For this review, take the finished solid that the model builds, in its own axes (mm). Face numbers are marked on the shaded views. A direction names the side the tool comes from. Coordinates: 2 decimals unless noted, no trailing zeros. Order: outer loops, then holes, each group sorted by start corner. A loop starts at its lowest first (then second) coordinate and runs counter-clockwise, first axis right, second up. Notation, with made-up numbers: (46.5, 30.25) -> (62.5, 30.25) arc R21 cw to (62.5, 51.25) -> close; hole circle Ø1 at (3, -19). An arc over 180 degrees is marked (long way). Return JSON: item names as keys, results as strings. Group by question number.
Item 1: Machinability: for the marked faces 5, 6 and 7, which of the approach directions +Z, -Z, +X, -X, +Y, -Y give a long, thin tool a straight path to every point of the face, cutting with its end or side? Answer none if there is none.
Item 2: Take a section at D-D (x = 6.25). Write out the cut boundary in (y, z).
Item 3: Take a section at B-B (y = 1.75). Write out the cut boundary in (x, z).
Item 4: Draft analysis for pull direction Z (two halves, no side actions). For the marked faces 1, 2, 3 and 4, state which applies: +Z half, -Z half, draft (parallel to the pull), parting line (faces both ways), or undercut.
Item 5: Insertion check: pin 1 (2.5 mm diameter, centred on y = 7.5, z = 8.5, fed in from -X); pin 2 (2 mm diameter, centred on y = 1.5, z = 13.5, fed in from -X); pin 3 (3 mm diameter, centred on x = 8, z = 10.5, fed in from +Y). Each pin has a flat end and moves straight along its axis. Give the tip position at first contact, or say it passes through.
Item 6: Take a section at C-C (z = 16). Write out the cut boundary in (x, y).
Item 7: For line 1 along Z through (x, y) = (0, 5.75); line 2 along X through (y, z) = (5.5, 9); line 3 along X through (y, z) = (6.5, 5), list the stretches that pass through material, from the lowest coordinate up.
Item 8: Take a section at A-A (z = 9). Write out the cut boundary in (x, y), then the cut area to 3 significant figures.
```python
from build123d import *

# Parameters (mm, degrees)
EXTRUDED_1_DEPTH = 18


with BuildPart() as part:
    # Эскиз1 → Extruded 1 (new body)
    with BuildSketch(Plane.XY):
        Polygon((-5, 0), (-9, 4), (-9, 6), (-5, 6), (-5, 9), (-0.25, 9), (0, 8.75), (0.25, 9), (5, 9), (5, 6), (9, 6), (9, 4), (5, 0), align=None)
    extrude(amount=EXTRUDED_1_DEPTH)

    # Эскиз2 → Revolved Cut 1 (revolve, cut)
    with BuildSketch(Plane(origin=(0, 0, 0), x_dir=(0, 0, -1), z_dir=(1, 0, 0))):
        Polygon((-9, 0), (-9, 9), (-5.6, 9), (-6.6, 8), (-6.6, 1), (-5.6, 0), align=None)
    revolve(axis=Axis((0, 0, 9), (0, 1, 0)), mode=Mode.SUBTRACT)


solid = part.part
```
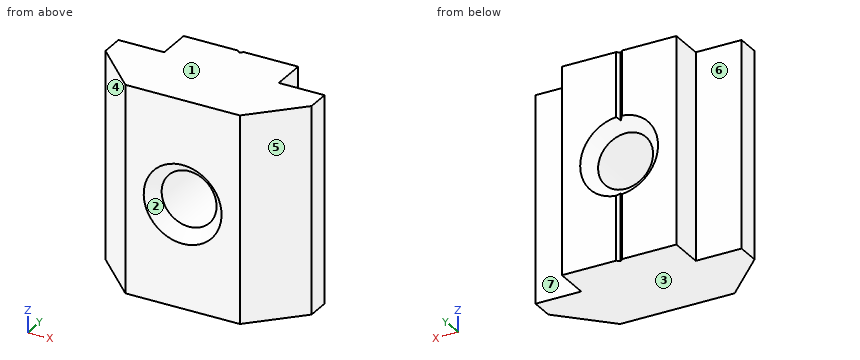
Findings below:
{
 "1": {"face 5": "+Z, -Z, +X, -Y", "face 6": "+Z, -Z, -X, +Y", "face 7": "+Z, -Z, +X, +Y"},
 "2": {"outline": "(1.25, 0) -> (6, 0) -> (6, 18) -> (1.25, 18) -> close"},
 "3": {"outline": "(-6.75, 0) -> (6.75, 0) -> (6.75, 18) -> (-6.75, 18) -> close; hole circle Ø4.8 at (0, 9)"},
 "4": {"face 1": "+Z half", "face 2": "undercut", "face 3": "-Z half", "face 4": "draft"},
 "5": {"pin 1": "stops at x = -5", "pin 2": "stops at x = -7.5", "pin 3": "stops at y = 6"},
 "6": {"outline": "(-9, 4) -> (-5, 0) -> (5, 0) -> (9, 4) -> (9, 6) -> (5, 6) -> (5, 9) -> (0.25, 9) -> (0, 8.75) -> (-0.25, 9) -> (-5, 9) -> (-5, 6) -> (-9, 6) -> close"},
 "7": {"line 1": "z = 0 to 6.6, 11.4 to 18", "line 2": "x = -9 to -2.4, 2.4 to 9", "line 3": "x = -5 to 5"},
 "8": {"outline": "(-9, 4) -> (-5, 0) -> (-3.4, 0) -> (-2.4, 1) -> (-2.4, 8) -> (-3.4, 9) -> (-5, 9) -> (-5, 6) -> (-9, 6) -> close; (2.4, 1) -> (3.4, 0) -> (5, 0) -> (9, 4) -> (9, 6) -> (5, 6) -> (5, 9) -> (3.4, 9) -> (2.4, 8) -> close", "area": "76.8 mm2"}
}
